For this review, take the finished solid that the model builds, in its own axes (mm). Round coordinates to 2 decimals unless told otherwise and drop trailing zeros. One line per item, written item: value. Start each with the question number.
Q1. For probe 1 along X at (y, z) = (-8, 474.5); probe 2 along Y at (x, z) = (0, 311); probe 3 along Y at (x, z) = (4.75, 232.5), list the stretches that pass through material, from the lowest coordinate up.
Q2. Add section A-A on z = 193. Give the number of separate pieces and of enclosed holes in the cut face, and give its area (3 significant figures).
Q3. Clearance check with flat-ended pins moving along their axes: pin 1 Ø0.8 at (y, z) = (1.5, 222) entering from +X; pin 2 Ø3 at (x, z) = (1, 159.5) entering from +Y; pin 3 Ø3 at (x, z) = (-1, 229.5) entering from -Y. State where each tip first meets the part, or that it passes through.
```python
from build123d import *

# Parameters (mm, degrees)
F0_R     = 2.1
F1_DEPTH = 505


with BuildPart() as f1:
    # F0 (on Top) → F1 (new body)
    with BuildSketch(Plane.XY):
        with BuildLine():
            Line((10, 4.64), (10, 8.5))
            ThreePointArc((10, 8.5), (9.56066, 9.56066), (8.5, 10))
            Line((8.5, 10), (4.64, 10))
            Line((4.64, 10), (2.84, 8.2))
            Line((2.84, 8.2), (5.49934, 8.2))
            Line((5.49934, 8.2), (5.49934, 6.56))
            Line((5.49934, 6.56), (2.84, 3.90066))
            Line((2.84, 3.90066), (0.25, 3.90066))
            Line((0.25, 3.90066), (0, 3.65066))
            Line((0, 3.65066), (-0.25, 3.90066))
            Line((-0.25, 3.90066), (-2.84, 3.90066))
            Line((-2.84, 3.90066), (-5.49934, 6.56))
            Line((-5.49934, 6.56), (-5.49934, 8.2))
            Line((-5.49934, 8.2), (-2.84, 8.2))
            Line((-2.84, 8.2), (-4.64, 10))
            Line((-4.64, 10), (-8.5, 10))
            ThreePointArc((-8.5, 10), (-9.56066, 9.56066), (-10, 8.5))
            Line((-10, 8.5), (-10, 4.64))
            Line((-10, 4.64), (-8.2, 2.84))
            Line((-8.2, 2.84), (-8.2, 5.49934))
            Line((-8.2, 5.49934), (-6.56, 5.49934))
            Line((-6.56, 5.49934), (-3.90066, 2.84))
            Line((-3.90066, 2.84), (-3.90066, 0.25))
            Line((-3.90066, 0.25), (-3.65066, 0))
            Line((-3.65066, 0), (-3.90066, -0.25))
            Line((-3.90066, -0.25), (-3.90066, -2.84))
            Line((-3.90066, -2.84), (-6.56, -5.49934))
            Line((-6.56, -5.49934), (-8.2, -5.49934))
            Line((-8.2, -5.49934), (-8.2, -2.84))
            Line((-8.2, -2.84), (-10, -4.64))
            Line((-10, -4.64), (-10, -8.5))
            ThreePointArc((-10, -8.5), (-9.56066, -9.56066), (-8.5, -10))
            Line((-8.5, -10), (-4.64, -10))
            Line((-4.64, -10), (-2.84, -8.2))
            Line((-2.84, -8.2), (-5.49934, -8.2))
            Line((-5.49934, -8.2), (-5.49934, -6.56))
            Line((-5.49934, -6.56), (-2.84, -3.90066))
            Line((-2.84, -3.90066), (-0.25, -3.90066))
            Line((-0.25, -3.90066), (0, -3.65066))
            Line((0, -3.65066), (0.25, -3.90066))
            Line((0.25, -3.90066), (2.84, -3.90066))
            Line((2.84, -3.90066), (5.49934, -6.56))
            Line((5.49934, -6.56), (5.49934, -8.2))
            Line((5.49934, -8.2), (2.84, -8.2))
            Line((2.84, -8.2), (4.64, -10))
            Line((4.64, -10), (8.5, -10))
            ThreePointArc((8.5, -10), (9.56066, -9.56066), (10, -8.5))
            Line((10, -8.5), (10, -4.64))
            Line((10, -4.64), (8.2, -2.84))
            Line((8.2, -2.84), (8.2, -5.49934))
            Line((8.2, -5.49934), (6.56, -5.49934))
            Line((6.56, -5.49934), (3.90066, -2.84))
            Line((3.90066, -2.84), (3.90066, -0.25))
            Line((3.90066, -0.25), (3.65066, 0))
            Line((3.65066, 0), (3.90066, 0.25))
            Line((3.90066, 0.25), (3.90066, 2.84))
            Line((3.90066, 2.84), (6.56, 5.49934))
            Line((6.56, 5.49934), (8.2, 5.49934))
            Line((8.2, 5.49934), (8.2, 2.84))
            Line((8.2, 2.84), (10, 4.64))
        make_face()
        Polygon((-6.56934, -7.63), (-6.56934, -8.2), (-8.2, -8.2), (-8.2, -6.56934), (-7.63, -6.56934), align=None, mode=Mode.SUBTRACT)
        Polygon((8.2, -8.2), (6.56934, -8.2), (6.56934, -7.63), (7.63, -6.56934), (8.2, -6.56934), align=None, mode=Mode.SUBTRACT)
        Polygon((-7.63, 6.56934), (-8.2, 6.56934), (-8.2, 8.2), (-6.56934, 8.2), (-6.56934, 7.63), align=None, mode=Mode.SUBTRACT)
        Circle(F0_R, mode=Mode.SUBTRACT)
        Polygon((6.56934, 7.63), (6.56934, 8.2), (8.2, 8.2), (8.2, 6.56934), (7.63, 6.56934), align=None, mode=Mode.SUBTRACT)
    extrude(amount=F1_DEPTH)


solid = f1.part
```
Result set:
1. probe 1: x = -10 to -8.2, -6.57 to -5.5, 5.5 to 6.57, 8.2 to 10
1. probe 2: y = -3.65 to -2.1, 2.1 to 3.65
1. probe 3: y = -10 to -8.2, -5.81 to -3.69, 3.69 to 5.81, 8.2 to 10
2. separate pieces: 1
2. enclosed holes: 5
2. area: 161 mm^2
3. pin 1: stops at x = 3.9
3. pin 2: stops at y = 3.9
3. pin 3: stops at y = -3.9
